Model file for the job. Use its own axes, mm. Face numbers are marked on the shaded views. A direction names the side the tool comes from. Give positions to 0.01 mm unless a question says otherwise; leave off trailing zeros. Order: outer loops, then holes, each group sorted by start corner. A loop starts at its lowest first (then second) coordinate and runs counter-clockwise, first axis right, second up. Notation, with made-up numbers: (79.25, 83.25) - (102.25, 83.25) arc R7 cw to (102.25, 92.25) - close; hole circle Ø3 at (-33.75, 62). An arc over 180 degrees is marked (long way). Use CSV: the item, a comma, the result in double quotes. Start each with the question number.
(1) Probe L1, parallel to X at y = -0.25, z = 9.5; L2, parallel to X at y = 0.5, z = 0.75; L3, parallel to X at y = -5, z = 7. List the from-to ranges inside material, lowest first.
(2) Pull direction X, two halves, no side cores. Call the marked faces 1, 2 and 3: +X half, -X half, draft (parallel to the pull), parting line (faces both ways), or undercut.
(3) Band-saw the part on D-D, the plane x = 9. Give the cut face in (y, z).
(4) Drop flat-ended pins along their axis: pin 1 Ø4 at (y, z) = (5.5, 4.5) entering from -X; pin 2 Ø1 at (y, z) = (0.5, 3.5) entering from -X; pin 3 Ø3 at (x, y) = (15, 0) entering from +Z; pin 4 Ø7 at (x, y) = (-3.5, -0.5) entering from -Z. Give the stop position or say it passes through.
(5) Band-saw the part on B-B, the plane z = 3.5. Give the cut face in (x, y).
(6) Tool access for the marked faces 4 and 5: list every direction of +Z, -Z, +X, -X, +Y, -Y with a clear straight run to the whole face (end or side of a thin tool).
(7) Band-saw the part on A-A, the plane x = 0. Give the cut face in (y, z) (3 decimals).
(8) Band-saw the part on C-C, the plane y = 7.75. Give the cut face in (x, z), then the cut area to 3 significant figures.
from build123d import *

# Parameters (mm, degrees)
SKETCH1_R           = 2.5
BOSS_EXTRUDE1_DEPTH = 10
SKETCH2_R           = 8.082903769
SKETCH2_R_2         = 6.625
BOSS_EXTRUDE3_DEPTH = 2.5
CHAMFER1_SIZE       = 1.5


with BuildPart() as part:
    # Sketch1 → Boss-Extrude1 (new body)
    with BuildSketch(Plane.XY):
        with BuildLine():
            Line((-5.2, -10.814804668), (-17.383333333, -4.956785473))
            ThreePointArc((-17.383333333, -4.956785473), (-20.5, 0), (-17.383333333, 4.956785473))
            Line((-17.383333333, 4.956785473), (-5.2, 10.814804668))
            ThreePointArc((-5.2, 10.814804668), (0, 12), (5.2, 10.814804668))
            Line((5.2, 10.814804668), (17.383333333, 4.956785473))
            ThreePointArc((17.383333333, 4.956785473), (20.5, 0), (17.383333333, -4.956785473))
            Line((17.383333333, -4.956785473), (5.2, -10.814804668))
            ThreePointArc((5.2, -10.814804668), (0, -12), (-5.2, -10.814804668))
        make_face()
        with Locations((-15, 0)):
            Circle(SKETCH1_R, mode=Mode.SUBTRACT)
        with Locations(Location((15, 0, 0), (0, 0, 180))):
            Circle(SKETCH1_R, mode=Mode.SUBTRACT)
        Polygon((8.082903769, 0), (4.041451884, 7), (-4.041451884, 7), (-8.082903769, 0), (-4.041451884, -7), (4.041451884, -7), align=None, mode=Mode.SUBTRACT)
    extrude(amount=BOSS_EXTRUDE1_DEPTH)

    # Sketch2 → Boss-Extrude3 (add)
    with BuildSketch(Plane.XY.offset(10)):
        Circle(SKETCH2_R)
        Circle(SKETCH2_R_2, mode=Mode.SUBTRACT)
    extrude(amount=-BOSS_EXTRUDE3_DEPTH)

    # Chamfer1
    chamfer1_edges = [part.edges().sort_by_distance(p)[0] for p in [
        (11.291666667, 7.88579507, 0),
        (20.5, 0, 0),
        (11.291666667, -7.88579507, 0),
        (0, -12, 0),
        (20.5, 0, 10),
        (11.291666667, 7.88579507, 10),
        (0, 12, 10),
        (-11.291666667, 7.88579507, 10),
        (-20.5, 0, 10),
        (6.062177826, -3.5, 0),
        (6.062177826, 3.5, 0),
        (0, 7, 0),
        (-6.062177826, 3.5, 0),
        (-6.062177826, -3.5, 0),
        (0, -7, 0),
        (-11.291666667, -7.88579507, 10),
        (0, -12, 10),
        (-11.291666667, -7.88579507, 0),
        (11.291666667, -7.88579507, 10),
        (-20.5, 0, 0),
        (-11.291666667, 7.88579507, 0),
        (0, 12, 0),
    ]]
    chamfer(chamfer1_edges, length=CHAMFER1_SIZE)


solid = part.part
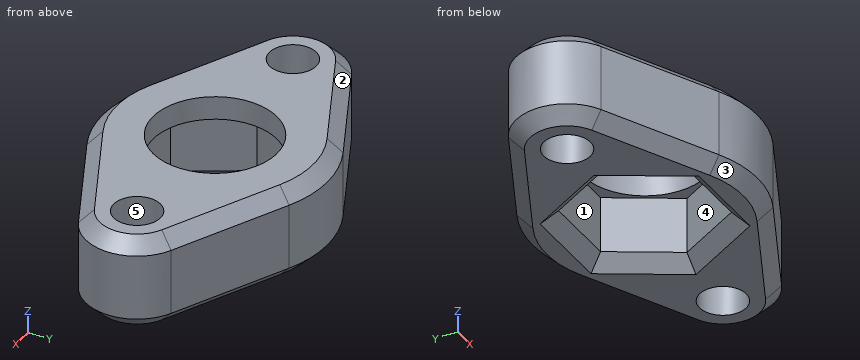
Answer block:
1,L1,"x = -19.49 to -17.49, -12.51 to -6.62, 6.62 to 12.51, 17.49 to 19.49"
1,L2,"x = -19.72 to -17.45, -12.55 to -8.66, 8.66 to 12.55, 17.45 to 19.72"
1,L3,"x = -17.29 to -5.2, 5.2 to 17.29"
2,face 1,"undercut"
2,face 2,"-X half"
2,face 3,"parting line"
3,outline,"(-8.99, 1.5) - (-7.32, 0) - (-1.41, 0) - (0, 0.71) - (1.41, 0) - (7.32, 0) - (8.99, 1.5) - (8.99, 8.5) - (7.32, 10) - (-7.32, 10) - (-8.99, 8.5) - close"
4,pin 1,"stops at x = -19.24"
4,pin 2,"stops at x = -20.5"
4,pin 3,"passes through"
4,pin 4,"stops at z = 7.5"
5,outline,"(-17.38, -4.96) - (-5.2, -10.81) arc R12 ccw to (5.2, -10.81) - (17.38, -4.96) arc R5.5 ccw to (17.38, 4.96) - (5.2, 10.81) arc R12 ccw to (-5.2, 10.81) - (-17.38, 4.96) arc R5.5 ccw to start; hole circle Ø5 at (-15, 0); hole (-8.08, 0) - (-4.04, -7) - (4.04, -7) - (8.08, 0) - (4.04, 7) - (-4.04, 7) - close; hole circle Ø5 at (15, 0)"
6,face 4,"-Z"
6,face 5,"+Z, -Z"
7,outline,"(-12, 1.5) - (-10.5, 0) - (-8.5, 0) - (-7, 1.5) - (-7, 7.5) - (-6.625, 7.5) - (-6.625, 10) - (-10.5, 10) - (-12, 8.5) - close; (6.625, 7.5) - (7, 7.5) - (7, 1.5) - (8.5, 0) - (10.5, 0) - (12, 1.5) - (12, 8.5) - (10.5, 10) - (6.625, 10) - close"
8,outline,"(-11.57, 1.5) - (-8.11, 0) - (-5.34, 0) - (-4.47, 0.75) - (4.47, 0.75) - (5.34, 0) - (8.11, 0) - (11.57, 1.5) - (11.57, 8.5) - (8.11, 10) - (-8.11, 10) - (-11.57, 8.5) - close"
8,area,"214 mm2"
